from build123d import *

# Parameters (mm, degrees)
F0_W      = 82.55
F0_H      = 98.425
F2_DEPTH  = 19.05
F3_R      = 3
F4_W      = 76.55
F4_H      = 13.05
F5_DEPTH  = 6.35
F6_W      = 36.55
F6_H      = 2.2
F7_DEPTH  = 2
F8_W      = 8.7
F8_H      = 2.2
F9_DEPTH  = 25
F10_W     = 6
F10_H     = 2.2
F11_DEPTH = 6.35
F12_SIZE  = 1.09999
F14_DEPTH = 0.5


# Not quite as in the source:
# - a fillet or chamfer is up to 0.001 mm smaller than in the source, because OpenCascade refuses the exact size


with BuildPart() as f2:
    # F0 (on Top) → F2 (new body)
    with BuildSketch(Plane.XY):
        with Locations((-41.275, 49.2125)):
            Rectangle(F0_W, F0_H)
    extrude(amount=-F2_DEPTH)

    # F3
    f3_edges = [f2.edges().sort_by_distance(p)[0] for p in [
        (-82.55, 49.2125, -19.05),
        (-82.55, 49.2125, 0),
        (0, 49.2125, 0),
        (0, 49.2125, -19.05),
    ]]
    fillet(f3_edges, radius=F3_R)

    # F4 (on face) → F5 (cut)
    with BuildSketch(Plane(origin=(0, 98.425, 0), x_dir=(-1, 0, 0), z_dir=(0, 1, 0))):
        with Locations((41.275, -9.525)):
            Rectangle(F4_W, F4_H)
    extrude(amount=-F5_DEPTH, mode=Mode.SUBTRACT)

    # F6 (on face) → F7 (cut)
    with BuildSketch(Plane(origin=(0, 92.075, 0), x_dir=(-1, 0, 0), z_dir=(0, 1, 0))):
        with Locations((41.275, -9.55)):
            Rectangle(F6_W, F6_H)
    extrude(amount=-F7_DEPTH, mode=Mode.SUBTRACT)

    # F8 (on face) → F9 (cut)
    with BuildSketch(Plane(origin=(0, 92.075, 0), x_dir=(-1, 0, 0), z_dir=(0, 1, 0))):
        with Locations((66.3, -9.55)):
            Rectangle(F8_W, F8_H)
        with Locations((16.25, -9.55)):
            Rectangle(F8_W, F8_H)
    extrude(amount=-F9_DEPTH, mode=Mode.SUBTRACT)

    # F10 (on face) → F11 (join, through all)
    with BuildSketch(Plane(origin=(0, 92.075, 0), x_dir=(-1, 0, 0), z_dir=(0, 1, 0))):
        with Locations((73.65, -9.55)):
            Rectangle(F10_W, F10_H)
        with Locations((8.9, -9.55)):
            Rectangle(F10_W, F10_H)
    extrude(amount=F11_DEPTH)

    # F12 (size 1.1 in the source; OpenCascade refuses exactly that, so slightly less here)
    f12_edges = [f2.edges().sort_by_distance(p)[0] for p in [
        (-8.9, 98.425, -8.45),
        (-8.9, 98.425, -10.65),
        (-73.65, 98.425, -8.45),
        (-73.65, 98.425, -10.65),
    ]]
    chamfer(f12_edges, length=F12_SIZE)

    # F13 (on face) → F14 (cut)
    with BuildSketch(Plane.XY):
        with BuildLine():
            Line((-6.7, 93.025), (-75.85, 93.025))
            ThreePointArc((-75.85, 93.025), (-77.617766953, 92.292766953), (-78.35, 90.525))
            Line((-78.35, 90.525), (-78.35, 6.8))
            ThreePointArc((-78.35, 6.8), (-77.617766953, 5.032233047), (-75.85, 4.3))
            Line((-75.85, 4.3), (-6.7, 4.3))
            ThreePointArc((-6.7, 4.3), (-4.932233047, 5.032233047), (-4.2, 6.8))
            Line((-4.2, 6.8), (-4.2, 90.525))
            ThreePointArc((-4.2, 90.525), (-4.932233047, 92.292766953), (-6.7, 93.025))
        make_face()
    extrude(amount=-F14_DEPTH, mode=Mode.SUBTRACT)


solid = f2.part
Model file for the job. Use its own axes, mm. A direction names the side the tool comes from. Give positions to 0.01 mm unless a question says otherwise; leave off trailing zeros. Order: outer loops, then holes, each group sorted by start corner. A loop starts at its lowest first (then second) coordinate and runs counter-clockwise, first axis right, second up. Notation, with made-up numbers: (-15.75, -21) - (26.25, -21) arc R24 cw to (26.25, -6) - close; hole circle Ø10 at (-30.5, 20.25). An arc over 180 degrees is marked (long way). One line per item, written item: value.
Item 1: Slice it at A-A (x = -54.5). List the corners of the cut face in (y, z) (3 decimals).
Response values:
outline: (0, -19.05) - (98.425, -19.05) - (98.425, -16.05) - (92.075, -16.05) - (92.075, -10.65) - (90.075, -10.65) - (90.075, -8.45) - (92.075, -8.45) - (92.075, -3) - (98.425, -3) - (98.425, 0) - (93.025, 0) - (93.025, -0.5) - (4.3, -0.5) - (4.3, 0) - (0, 0) - close
Item 2: Slice it at D-D (z = -7.25). List the corners of the cut face in (x, y) (3 decimals).
Response values:
outline: (-82.55, 0) - (0, 0) - (0, 98.425) - (-3, 98.425) - (-3, 92.075) - (-79.55, 92.075) - (-79.55, 98.425) - (-82.55, 98.425) - close
Item 3: Wall check: line 1 (Z direction, x = -25.5, y = 91); line 2 (Z direction, x = -60, y = 39); line 3 (Z direction, x = -59, y = 94). Give the ranges that are in metal, low to high.
Response values:
line 1: -19.05 to -10.65, -8.45 to -0.5
line 2: -19.05 to -0.5
line 3: -19.05 to -16.05, -3 to 0
Item 4: Slice it at B-B (y = 87.5). List the corners of the cut face in (x, z), then the cut area to 3 significant figures.
Response values:
outline: (-82.55, -16.05) arc R3 ccw to (-79.55, -19.05) - (-3, -19.05) arc R3 ccw to (0, -16.05) - (0, -3) arc R3 ccw to (-3, 0) - (-4.2, 0) - (-4.2, -0.5) - (-78.35, -0.5) - (-78.35, 0) - (-79.55, 0) arc R3 ccw to (-82.55, -3) - close; hole (-70.65, -10.65) - (-61.95, -10.65) - (-61.95, -8.45) - (-70.65, -8.45) - close; hole (-20.6, -10.65) - (-11.9, -10.65) - (-11.9, -8.45) - (-20.6, -8.45) - close
area: 1,490 mm2
Item 5: Pin check, flat tips, straight feed: pin 1 Ø2.5 at (x, y) = (-15, 84) entering from +Z; pin 2 Ø1.8 at (x, z) = (-68, -9.5) entering from +Y (3 decimals). Stop position of each tip, or through.
Response values:
pin 1: z = -0.5
pin 2: y = 67.075
Item 6: Two-plate mould, pull along X, no slides. Class faces 1 (the flat face through (-82.55, 49, -9)), 2 (the flat face through (-16, 80, -10.65)), 3 (the cylindrical face through (-0.86, 49.9, -18.15)): released by +X, released by -X, zero draft, split by the parting line, or undercut.
Response values:
face 1: released by -X
face 2: undercut
face 3: released by +X
Item 7: Slice it at C-C (y = 50). List the corners of the cut face in (x, z).
Response values:
outline: (-82.55, -16.05) arc R3 ccw to (-79.55, -19.05) - (-3, -19.05) arc R3 ccw to (0, -16.05) - (0, -3) arc R3 ccw to (-3, 0) - (-4.2, 0) - (-4.2, -0.5) - (-78.35, -0.5) - (-78.35, 0) - (-79.55, 0) arc R3 ccw to (-82.55, -3) - close
Item 8: Tool access for faces 4 (the flat face through (-42, 0, -9)), 5 (the flat face through (-74, 95, -10.65)), 6 (the cylindrical face through (-4.952, 5.013, -0.246)): list every direction of +Z, -Z, +X, -X, +Y, -Y with a clear straight run to the whole face (end or side of a thin tool).
Response values:
face 4: +Z, -Z, +X, -X, -Y
face 5: +Y
face 6: +Z
